from build123d import *

# Parameters (mm, degrees)
F1_DEPTH = 76.708
F3_DEPTH = 88.392


with BuildPart() as f1:
    # F0 (on Right) → F1 (new body)
    with BuildSketch(Plane.YZ):
        Polygon((32.097038, 35.508316), (-51.324245, 35.508316), (-51.324245, -38.609475), (33.337504, -38.609475), (33.337504, 31.166688), align=None)
    extrude(amount=F1_DEPTH)

    # F2 (on face) → F3 (cut)
    with BuildSketch(Plane.XZ.offset(51.324245)):
        Polygon((76.708, 35.508316), (26.148705, 35.508316), (54.679401, -7.597849), (76.708, -7.597849), align=None)
    extrude(amount=-F3_DEPTH, mode=Mode.SUBTRACT)


solid = f1.part
The model under review builds one solid part; all positions refer to its coordinate system, in mm. A direction names the side the tool comes from. Round coordinates to 2 decimals unless told otherwise and drop trailing zeros. Order: outer loops, then holes, each group sorted by start corner. A loop starts at its lowest first (then second) coordinate and runs counter-clockwise, first axis right, second up. Notation, with made-up numbers: (-25, 9.5) -> (-6, 9.5) arc R30 ccw to (-6, 44.5) -> close; hole circle Ø4 at (-20.75, 18). An arc over 180 degrees is marked (long way). Use CSV: the item, a comma, the result in double quotes. Start each with the question number.
(1) Wall thickness on probe 1 along Z at (x, y) = (64.5, 21.5); probe 2 along Z at (x, y) = (27, -38); probe 3 along X at (y, z) = (7.5, 22): over which ranges is each line inside the solid? List them lowest first. Write a range as from..to.
(2) Consider section C-C on z = 29. Write out the cut boundary in (x, y).
(3) Tool access review of faces 1 (the face through (66, -10, -7.598)), 2 (the face through (76.708, -10, -23)): name each direction out of +Z, -Z, +X, -X, +Y, -Y from which nothing blocks a thin tool from reaching the whole face with its end or side.
(4) Insertion check: pin 1 (3 mm diameter, centred on x = 57.5, y = -13.5, fed in from +Z); pin 2 (1.5 mm diameter, centred on x = 34, y = -11, fed in from +Z); pin 3 (10 mm diameter, centred on x = 45, y = 20.5, fed in from +Z). Each pin has a flat end and moves straight along its axis. Give the tip position at first contact, or say it passes through.
(5) Consider section B-B on x = 65.5. Write out the cut boundary in (y, z), and give its area (3 significant figures).
(6) Consider section A-A on y = -34.5. Write out the cut boundary in (x, z), and give its area (3 significant figures).
Responses:
1,probe 1,"-38.61..-7.6"
1,probe 2,"-38.61..34.22"
1,probe 3,"0..35.09"
2,outline,"(0, -51.32) -> (30.46, -51.32) -> (30.46, 33.34) -> (0, 33.34) -> close"
3,face 1,"+Z, +X, +Y, -Y"
3,face 2,"+Z, -Z, +X, +Y, -Y"
4,pin 1,"z = -7.6"
4,pin 2,"z = 24.78"
4,pin 3,"z = 14.58"
5,outline,"(-51.32, -38.61) -> (33.34, -38.61) -> (33.34, -7.6) -> (-51.32, -7.6) -> close"
5,area,"2,630 mm²"
6,outline,"(0, -38.61) -> (76.71, -38.61) -> (76.71, -7.6) -> (54.68, -7.6) -> (26.15, 35.51) -> (0, 35.51) -> close"
6,area,"4,120 mm²"
